CAD build for the part. Positions are in the model's coordinates, mm. Give positions to 0.01 mm unless a question says otherwise; leave off trailing zeros. Write each loop counter-clockwise with the first axis right and the second up, starting at its lowest first coordinate (ties: lowest second). Pieces come first, ordered by that corner, then holes. Notation, with made-up numbers: (0.5, 38.5) - (29.5, 38.5) arc R16 cw to (29.5, 65.5) - close; hole circle Ø10 at (32, 20.25). An arc over 180 degrees is marked (long way). Put each result on its own line as item: value. Start each with the question number.
1. Cut at A-A on y = 0. List the corners of the cut face in (x, z), and give its area (3 significant figures).
2. Drop flat-ended pins along their axis: pin 1 (2 mm diameter, centred on x = -6, z = 4.5, fed in from -Y); pin 2 (2 mm diameter, centred on x = 2.5, y = -9, fed in from +Z); pin 3 (5 mm diameter, centred on y = 6.5, z = 7, fed in from +X). Give the stop position or say it passes through.
3. Cut at C-C on z = 7.5. List the corners of the cut face in (x, y).
4. Mould opens along Y. For faces 1 (the cylindrical face through (-14.985, -0.66, 4.958)), 2 (the cylindrical face through (-2.17, 9.76, 4.44)), 3 (the flat face through (7, -8, 0)) say: +Y half, -Y half, draft (parallel to the pull), parting line (faces both ways), or undercut.
5. Wall check: line 1 (Y direction, x = 0, z = 2); line 2 (X direction, y = 1.5, z = 4.5); line 3 (X direction, y = 5.75, z = 5). Give the ranges that are in metal, low to high.
Autodesk Fusion 360 part; units mm, degrees
sketch "Esquisse1" plane through (0, 0, 0) normal (0, 0, 1) x (1, 0, 0)
  circle A0 centre (0, 0) radius 10
  circle A1 centre (0, 0) radius 15
  dimension "d1" = 20
  dimension "d2" = 30
extrude "Extrusion1" add sketch "Esquisse1" along normal blind 10
fillet "Congé1" radius 2 2 edges at (-13.9849, -5.4242, 10) (-13.9849, -5.4242, 0)
chamfer "Chanfrein1" distance 1 angle 45 1 edges at (-9.3233, 3.6162, 10)
Report:
1. outline: (-15, 2) arc R2 ccw to (-13, 0) - (-10, 0) - (-10, 9) - (-11, 10) - (-13, 10) arc R2 ccw to (-15, 8) - close; (10, 0) - (13, 0) arc R2 ccw to (15, 2) - (15, 8) arc R2 ccw to (13, 10) - (11, 10) - (10, 9) - close
1. area: 95.6 mm²
2. pin 1: stops at y = -14.14
2. pin 2: stops at z = 9.34
2. pin 3: stops at x = 14.46
3. outline: circle Ø30 at (0, 0); hole circle Ø20 at (0, 0)
4. face 1: parting line
4. face 2: undercut
4. face 3: draft
5. line 1: y = -15 to -10, 10 to 15
5. line 2: x = -14.92 to -9.89, 9.89 to 14.92
5. line 3: x = -13.85 to -8.18, 8.18 to 13.85
